Part model, mm, in its own coordinate system. A direction names the side the tool comes from. Give positions to 0.01 mm unless a question says otherwise; leave off trailing zeros. Order: outer loops, then holes, each group sorted by start corner. A loop starts at its lowest first (then second) coordinate and runs counter-clockwise, first axis right, second up. Notation, with made-up numbers: M -5,9 L 31,9 A13 cw 31,32 Z; hole C -7,63 d8. An arc over 180 degrees is marked long. Return JSON: item names as keys, results as strings.
from build123d import *

# Parameters (mm, degrees)
F0_W         = 62
F0_H         = 91
F1_DEPTH     = 3
F2_W         = 62
F2_H         = 91
F2_W_2       = 57
F2_H_2       = 86
F3_DEPTH     = 30
F4_R         = 3.5
F5_DEPTH     = 5
F6_R         = 2.4
F7_DEPTH     = 3
F8_W         = 57
F8_H         = 25
F9_DEPTH     = 2.5
F10_W        = 18
F10_H        = 8
F10_R        = 3.5
F11_DEPTH    = 2.5
F12_DEPTH    = 7
F13_W        = 42
F13_H        = 7.5
F14_DEPTH    = 8
F15_R        = 2.4
F16_DEPTH    = 3
F17_W        = 11
F17_H        = 7.5
F18_DEPTH    = 1.8
F19_R        = 1
F20_R        = 3.5
F21_DEPTH    = 2
F22_T1_DEPTH = 62
F22_T3_DEPTH = 91
F24_DEPTH    = 33
F25_R        = 2.05
F25_R_2      = 1.7907732373
F26_DEPTH    = 4
F28_DEPTH    = 19


# Not quite as in the source:
# - a fillet or chamfer that OpenCascade refuses, or shapes differently, is made with other operations: its cross-section is extruded or revolved along the edge and cut away or added


with BuildPart() as f1:
    # F0 (on Top) → F1 (new body)
    with BuildSketch(Plane.XY):
        Rectangle(F0_W, F0_H)
    extrude(amount=F1_DEPTH)

    # F2 (on face) → F3 (join)
    with BuildSketch(Plane.XY.offset(3)):
        Rectangle(F2_W, F2_H)
        Rectangle(F2_W_2, F2_H_2, mode=Mode.SUBTRACT)
    extrude(amount=F3_DEPTH)

    # F4 (on face) → F5 (join)
    with BuildSketch(Plane.XY.offset(3)):
        with Locations((-24.5, 39)):
            Circle(F4_R)
        with Locations((24.5, 39)):
            Circle(F4_R)
        with Locations((-24.5, -19)):
            Circle(F4_R)
        with Locations((24.5, -19)):
            Circle(F4_R)
    extrude(amount=F5_DEPTH)

    # F6 (on face) → F7 (cut)
    with BuildSketch(Plane.XY.offset(8)):
        with Locations((-24.5, 39)):
            Circle(F6_R)
        with Locations((24.5, 39)):
            Circle(F6_R)
        with Locations((-24.5, -19)):
            Circle(F6_R)
        with Locations((24.5, -19)):
            Circle(F6_R)
    extrude(amount=-F7_DEPTH, mode=Mode.SUBTRACT)

    # F8 (on face) → F9 (cut, through all)
    with BuildSketch(Plane.XZ.offset(45.5)):
        with Locations((0, 20.5)):
            Rectangle(F8_W, F8_H)
    extrude(amount=-F9_DEPTH, mode=Mode.SUBTRACT)

    # F10 (on face) → F11 (cut, through all)
    with BuildSketch(Plane.YZ.offset(-28.5)):
        Polygon((26.9, 9), (36.9, 9), (36.9, 14), (31.9, 14), (26.9, 14), align=None)
        with Locations((10.5, 13)):
            Rectangle(F10_W, F10_H)
        with Locations((-11, 12.9)):
            Circle(F10_R)
    extrude(amount=-F11_DEPTH, mode=Mode.SUBTRACT)

    # F12 (add): a face of the model
    f12_faces = [f1.faces().sort_by_distance(p)[0] for p in [
        (0, 45.5, 16.5),
    ]]
    extrude(f12_faces, amount=F12_DEPTH)

    # F13 (on face) → F14 (cut)
    with BuildSketch(Plane.XY.offset(33)):
        with Locations((0, 46.75)):
            Rectangle(F13_W, F13_H)
    extrude(amount=-F14_DEPTH, mode=Mode.SUBTRACT)

    # F15 (on face) → F16 (cut)
    with BuildSketch(Plane.XY.offset(25)):
        with Locations((-15, 46.6)):
            Circle(F15_R)
        with Locations((15, 46.6)):
            Circle(F15_R)
    extrude(amount=-F16_DEPTH, mode=Mode.SUBTRACT)

    # F17 (on face) → F18 (cut)
    with BuildSketch(Plane.XY.offset(25)):
        with Locations((-6.5, 46.75)):
            Rectangle(F17_W, F17_H)
    extrude(amount=-F18_DEPTH, mode=Mode.SUBTRACT)

    # F19
    f19_edges = [f1.edges().sort_by_distance(p)[0] for p in [
        (-12, 46.75, 23.2),
        (-1, 46.75, 23.2),
    ]]
    fillet(f19_edges, radius=F19_R)

    # F20 (on face) → F21 (cut, through all)
    with BuildSketch(Plane.XZ.offset(-50.5)):
        with Locations((-6.5, 28.5)):
            Circle(F20_R)
    extrude(amount=-F21_DEPTH, mode=Mode.SUBTRACT)

    # F22: fillet of radius 1 on 8 edges, made by hand

    # F22_s2 → F22_t1 (join)
    with BuildSketch(Plane.YZ.offset(-31)):
        with BuildLine():
            ThreePointArc((43, 4), (42.7071067812, 3.2928932188), (42, 3))
            Line((42, 3), (43, 3))
            Line((43, 3), (43, 4))
        make_face()
        with BuildLine():
            ThreePointArc((-42, 3), (-42.7071067812, 3.2928932188), (-43, 4))
            Line((-43, 4), (-43, 3))
            Line((-43, 3), (-42, 3))
        make_face()
    extrude(amount=F22_T1_DEPTH)

    # F22_s4 → F22_t3 (join)
    with BuildSketch(Plane.XZ.offset(-45.5)):
        with BuildLine():
            ThreePointArc((-27.5, 3), (-28.2071067812, 3.2928932188), (-28.5, 4))
            Line((-28.5, 4), (-28.5, 3))
            Line((-28.5, 3), (-27.5, 3))
        make_face()
        with BuildLine():
            ThreePointArc((28.5, 4), (28.2071067812, 3.2928932188), (27.5, 3))
            Line((27.5, 3), (28.5, 3))
            Line((28.5, 3), (28.5, 4))
        make_face()
    extrude(amount=F22_T3_DEPTH)

    # F22_s5 → F22_t6 (revolve)
    with BuildSketch(Plane.XZ.offset(-39)):
        with BuildLine():
            ThreePointArc((29, 3), (28.2928932188, 3.2928932188), (28, 4))
            Line((28, 4), (28, 3))
            Line((28, 3), (29, 3))
        make_face()
    revolve(axis=Axis((24.5, 39, 3), (0, 0, 1)))

    # F22_s7 → F22_t8 (revolve)
    with BuildSketch(Plane.XZ.offset(-39)):
        with BuildLine():
            ThreePointArc((-20, 3), (-20.7071067812, 3.2928932188), (-21, 4))
            Line((-21, 4), (-21, 3))
            Line((-21, 3), (-20, 3))
        make_face()
    revolve(axis=Axis((-24.5, 39, 3), (0, 0, 1)))

    # F22_s9 → F22_t10 (revolve)
    with BuildSketch(Plane.XZ.offset(19)):
        with BuildLine():
            ThreePointArc((-20, 3), (-20.7071067812, 3.2928932188), (-21, 4))
            Line((-21, 4), (-21, 3))
            Line((-21, 3), (-20, 3))
        make_face()
    revolve(axis=Axis((-24.5, -19, 3), (0, 0, 1)))

    # F22_s11 → F22_t12 (revolve)
    with BuildSketch(Plane.XZ.offset(19)):
        with BuildLine():
            ThreePointArc((29, 3), (28.2928932188, 3.2928932188), (28, 4))
            Line((28, 4), (28, 3))
            Line((28, 3), (29, 3))
        make_face()
    revolve(axis=Axis((24.5, -19, 3), (0, 0, 1)))

    # F23 (on face) → F24 (join, through all)
    with BuildSketch(Plane.XY):
        with BuildLine():
            Line((31, -45.5), (32.5, -45.5))
            ThreePointArc((32.5, -45.5), (35.25, -42.75), (32.5, -40))
            Line((32.5, -40), (31, -40))
            Line((31, -40), (31, -45.5))
        make_face()
        with BuildLine():
            Line((-31, -40), (-32.5, -40))
            ThreePointArc((-32.5, -40), (-35.25, -42.75), (-32.5, -45.5))
            Line((-32.5, -45.5), (-31, -45.5))
            Line((-31, -45.5), (-31, -40))
        make_face()
        with BuildLine():
            Line((-31, 52.5), (-33.75, 52.5))
            ThreePointArc((-33.75, 52.5), (-36.5, 49.75), (-33.75, 47))
            Line((-33.75, 47), (-31, 47))
            Line((-31, 47), (-31, 52.5))
        make_face()
        with BuildLine():
            Line((31, 47), (33.75, 47))
            ThreePointArc((33.75, 47), (36.5, 49.75), (33.75, 52.5))
            Line((33.75, 52.5), (31, 52.5))
            Line((31, 52.5), (31, 47))
        make_face()
    extrude(amount=F24_DEPTH)

    # F25 (on face) → F26 (cut)
    with BuildSketch(Plane.XY.offset(33)):
        with Locations((-32.5, -42.75)):
            Circle(F25_R)
        with Locations((32.5, -42.75)):
            Circle(F25_R)
        with Locations((-33.75, 49.75)):
            Circle(F25_R_2)
        with Locations((33.75, 49.75)):
            Circle(F25_R)
    extrude(amount=-F26_DEPTH, mode=Mode.SUBTRACT)

    # F27 (on face) → F28 (cut, through all)
    with BuildSketch(Plane.XY.offset(25)):
        Polygon((-8, 43), (8, 43), (8, 47), (0, 47), (-8, 47), align=None)
    extrude(amount=-F28_DEPTH, mode=Mode.SUBTRACT)


solid = f1.part
Q1. Pin check, flat tips, straight feed: pin 1 (1.5 mm diameter, centred on x = -17, y = 11, fed in from +Z); pin 2 (10 mm diameter, centred on y = 9.5, z = 14, fed in from +X); pin 3 (12 mm diameter, centred on y = 8, z = 10.5, fed in from -X). Stop position of each tip, or through.
Established:
{"pin 1": "stops at z = 3", "pin 2": "stops at x = 31", "pin 3": "stops at x = -31"}
Q2. Band-saw the part on D-D (z = 27). Give the cut face in (x, y).
Established:
{"outline": "M -33.75,47 L -31,47 L -31,-40 L -32.5,-40 A2.75 ccw -32.5,-45.5 L -28.5,-45.5 L -28.5,43 L -21,43 L -21,50.5 L -9.66,50.5 L -9.66,52.5 L -33.75,52.5 A2.75 ccw Z; M -3.34,50.5 L 21,50.5 L 21,43 L 28.5,43 L 28.5,-45.5 L 32.5,-45.5 A2.75 ccw 32.5,-40 L 31,-40 L 31,47 L 33.75,47 A2.75 ccw 33.75,52.5 L -3.34,52.5 Z"}
Q3. Two-plate mould, pull along Z, no slides. Class faces 1 (the flat face through (0, -44, 8)), 2 (the flat face through (0, 50.5, 29)), 3 (the flat face through (-30, 26.9, 12)): +Z half, -Z half, draft (parallel to the pull), parting line (faces both ways), or undercut.
Established:
{"face 1": "+Z half", "face 2": "draft", "face 3": "undercut"}
Q4. Band-saw the part on C-C (x = -15). Give the cut face in (y, z), then the cut area to 3 significant figures.
Established:
{"outline": "M -45.5,0 L 52.5,0 L 52.5,33 L 50.5,33 L 50.5,25 L 49,25 L 49,22 L 44.2,22 L 44.2,25 L 43,25 L 43,4 A1 cw 42,3 L -42,3 A1 cw -43,4 L -43,8 L -45.5,8 Z", "area": "518 mm²"}
Q5. Band-saw the part on A-A (y = 17.5). Give the cut face in (x, z).
Established:
{"outline": "M -31,0 L 31,0 L 31,33 L 28.5,33 L 28.5,4 A1 cw 27.5,3 L -27.5,3 A1 cw -28.5,4 L -28.5,9 L -31,9 Z; M -31,17 L -28.5,17 L -28.5,33 L -31,33 Z"}
Q6. Probe line 1 along Y through (x, z) = (-15, 22.8); line 2 along Y through (x, z) = (-33.75, 30.4); line 3 along X through (y, z) = (17.5, 30). List the from-to ranges inside material, lowest first.
Established:
{"line 1": "y = 43 to 44.2, 49 to 52.5", "line 2": "y = -45.2 to -44.37, -41.13 to -40.3, 47 to 47.96, 51.54 to 52.5", "line 3": "x = -31 to -28.5, 28.5 to 31"}
Q7. 3-axis set-ups, long thin cutter, end or side, ignore diameter. For faces 4 (the flat face through (15, 47, 22)), 5 (the cylindrical face through (-29.732, -11.759, 9.483)), 6 (the flat face through (27, -18, 8)), 7 (the flat face through (-31, 3, 20)): which of +Z, -Z, +X, -X, +Y, -Y reach the whole face in a straight line?
Established:
{"face 4": "+Z", "face 5": "-X", "face 6": "+Z, -Y", "face 7": "+Z, -Z, -X"}
Q8. Band-saw the part on B-B (z = 12.9). Give the number of separate pieces and of enclosed holes in the cut face, then the cut area to 3 significant figures.
Established:
{"separate pieces": "4", "enclosed holes": "0", "area": "974 mm²"}
